Read the model definition and answer for the solid it produces. Units are mm, in the model's axes. A direction names the side the tool comes from. Coordinates: 2 decimals unless noted, no trailing zeros. Order: outer loops, then holes, each group sorted by start corner. A loop starts at its lowest first (then second) coordinate and runs counter-clockwise, first axis right, second up. Notation, with made-up numbers: (-26.75, 12) - (-7.75, 12) arc R27 cw to (-7.75, 31) - close; hole circle Ø7 at (77.25, -11). An arc over 180 degrees is marked (long way). Use one line per item in the form item = value.
```python
from build123d import *

# Parameters (mm, degrees)
BOSS_EXTRUDE1_DEPTH      = 10
SKETCH3_R                = 6.5
SKETCH3_R_2              = 4
BOSS_EXTRUDE3_DEPTH      = 7.5
SKETCH7_W                = 15
SKETCH7_H                = 12.050233058
BOSS_EXTRUDE4_DEPTH      = 10
BOSS_EXTRUDE5_DEPTH      = 10
BOSS_EXTRUDE5_DEPTH_BACK = 10
SKETCH9_R                = 6.726812024
SKETCH9_R_2              = 4.5
FILLET1_R                = 10
FILLET2_R                = 10
FILLET3_R                = 10
FILLET4_R                = 10


with BuildPart() as part:
    # Sketch1 → Boss-Extrude1 (new body)
    with BuildSketch(Plane(origin=(0, 0, 0), x_dir=(1, 0, 0), z_dir=(0, 1, 0))):
        Polygon((-11.814153955, -17.668422436), (-29.581045004, -26.851971991), (-59, -113), (-73.793817424, -113), (-41.477337097, -18.36709911), (-5.943554998, 0), (5.943554998, 0), (41.477337097, -18.36709911), (73.793817424, -113), (59, -113), (29.581045004, -26.851971991), (11.814153955, -17.668422436), align=None)
    extrude(amount=BOSS_EXTRUDE1_DEPTH)

    # Sketch3 → Boss-Extrude3 (add, symmetric)
    with BuildSketch(Plane(origin=(-66.396908712, 0, 0), x_dir=(0, 0, -1), z_dir=(1, 0, 0))):
        with Locations((-117.153311931, 5)):
            Circle(SKETCH3_R)
        with Locations((-117.153311931, 5)):
            Circle(SKETCH3_R_2, mode=Mode.SUBTRACT)
    boss_extrude3 = extrude(amount=BOSS_EXTRUDE3_DEPTH, both=True)

    # Mirror3: Boss-Extrude3 across plane
    add(boss_extrude3.mirror(Plane(origin=(0, 0, 0), x_dir=(0, 0, 1), z_dir=(1, 0, 0))))

    # Sketch7 → Boss-Extrude4 (add)
    with BuildSketch(Plane(origin=(0, 10, 0), x_dir=(1, 0, 0), z_dir=(0, 1, 0))):
        with Locations((0, 6.025116529)):
            Rectangle(SKETCH7_W, SKETCH7_H)
    extrude(amount=-BOSS_EXTRUDE4_DEPTH)

    # Sketch9 → Boss-Extrude5 (add, two sides: drawn at the far end of the back side and taken through both)
    with BuildSketch(Plane(origin=(0, 0, 0), x_dir=(0, 0, -1), z_dir=(1, 0, 0)).offset(-BOSS_EXTRUDE5_DEPTH_BACK)):
        with Locations((16.550233058, 5)):
            Circle(SKETCH9_R)
        with Locations((16.550233058, 5)):
            Circle(SKETCH9_R_2, mode=Mode.SUBTRACT)
    extrude(amount=BOSS_EXTRUDE5_DEPTH + BOSS_EXTRUDE5_DEPTH_BACK)

    # Fillet1
    # the kernel refuses this fillet: 10 mm, written as the material it adds along each edge
    with BuildSketch(Plane(origin=(-5.943554998, 0, 0), x_dir=(-0.88834455248328, 0, 0.4591774777504672), z_dir=(0, 1, 0))) as fillet1_piece_1:
        with BuildLine():
            CenterArc((5.095194407, -10), FILLET1_R, 90, 21.792944461)
            Line((1.382659439, -0.71468449), (0, 0))
            Line((0, 0), (5.095194407, 0))
        make_face()
    extrude(amount=10)

    # Fillet2
    # the kernel refuses this fillet: 10 mm, written as the material it adds along each edge
    with BuildSketch(Plane(origin=(5.943554998, 0, 0), x_dir=(0.8883445524832799, 0, 0.4591774777504676), z_dir=(0, 1, 0))) as fillet2_piece_1:
        with BuildLine():
            CenterArc((5.095194407, 10), FILLET2_R, 248.207055539, 21.792944461)
            Line((1.382659439, 0.71468449), (0, 0))
            Line((0, 0), (5.095194407, 0))
        make_face()
    extrude(amount=10)

    # Fillet3
    # the kernel refuses this fillet: 10 mm, written as the material it adds along each edge
    with BuildSketch(Plane(origin=(11.814153955, 0, 17.668422436), x_dir=(0.8883445524832799, 0, 0.4591774777504676), z_dir=(0, 1, 0)), Plane(origin=(-11.814153955, 0, 17.668422436), x_dir=(1, 0, 0), z_dir=(0, 1, 0))) as fillet3_piece_1:
        with BuildLine():
            CenterArc((FILLET3_R * 0.243164033357, -FILLET3_R), FILLET3_R, 90, 27.334044372)
            Line((-FILLET3_R * 0.216013444393, -FILLET3_R * 0.111655447517), (0, 0))
            Line((0, 0), (FILLET3_R * 0.243164033357, 0))
        make_face()
    extrude(amount=10)
    with BuildSketch(Plane(origin=(29.581045004, 0, 26.851971991), x_dir=(0.3231689910588884, 0, 0.946341272067313), z_dir=(0, 1, 0)), Plane(origin=(-29.581045004, 0, 26.851971991), x_dir=(0.8883445524832806, 0, -0.4591774777504663), z_dir=(0, 1, 0))) as fillet3_piece_2:
        with BuildLine():
            CenterArc((FILLET3_R * 0.402111719604, -FILLET3_R), FILLET3_R, 90, 43.811274916)
            Line((-FILLET3_R * 0.290173472026, -FILLET3_R * 0.278375988862), (0, 0))
            Line((0, 0), (FILLET3_R * 0.402111719604, 0))
        make_face()
    extrude(amount=10)
    with BuildSketch(Plane(origin=(-52.198620973, 10, 113), x_dir=(0, 0, -1), z_dir=(-1, 0, 0))) as fillet3_piece_3_section:
        with BuildLine():
            CenterArc((2.720551611, -10), FILLET3_R, 90, 24.619977329)
            ThreePointArc((-1.445426294, -0.909090909), (-0.692731114, -0.502215954), (0, 0))
            Line((0, 0), (2.720551611, 0))
        make_face()
    fillet3_piece_3 = extrude(amount=28.396575479, mode=Mode.PRIVATE)
    fillet3_piece_3 = split(fillet3_piece_3, bisect_by=Plane(origin=(-58.289676239, 10, 110.919946807), z_dir=(-0.9463412720673133, 0, -0.3231689910588876)), keep=Keep.TOP, mode=Mode.PRIVATE)
    fillet3_piece_3 = split(fillet3_piece_3, bisect_by=Plane(origin=(-71.538454048, 10, 106.395580932), z_dir=(0.9463412720673133, 0, 0.3231689910588875)), keep=Keep.TOP, mode=Mode.PRIVATE)
    fillet3_piece_3 = split(fillet3_piece_3, bisect_by=Plane(origin=(-73.896908712, 10, 113), z_dir=(1, 0, 0)), keep=Keep.TOP, mode=Mode.PRIVATE)
    add(fillet3_piece_3)
    with BuildSketch(Plane(origin=(80.595196452, 10, 113), x_dir=(0, 0, -1), z_dir=(-1, 0, 0))) as fillet3_piece_4_section:
        with BuildLine():
            CenterArc((2.720551611, -10), FILLET3_R, 90, 24.619977329)
            ThreePointArc((-1.445426294, -0.909090909), (-0.692731114, -0.502215954), (0, 0))
            Line((0, 0), (2.720551611, 0))
        make_face()
    fillet3_piece_4 = extrude(amount=28.396575479, mode=Mode.PRIVATE)
    fillet3_piece_4 = split(fillet3_piece_4, bisect_by=Plane(origin=(74.504141186, 10, 115.080053193), z_dir=(-0.9463412720673132, 0, 0.32316899105888797)), keep=Keep.TOP, mode=Mode.PRIVATE)
    fillet3_piece_4 = split(fillet3_piece_4, bisect_by=Plane(origin=(61.255363377, 10, 119.604419068), z_dir=(0.9463412720673132, 0, -0.32316899105888797)), keep=Keep.TOP, mode=Mode.PRIVATE)
    fillet3_piece_4 = split(fillet3_piece_4, bisect_by=Plane(origin=(73.896908712, 10, 113), z_dir=(-1, 0, 0)), keep=Keep.TOP, mode=Mode.PRIVATE)
    add(fillet3_piece_4)
    with BuildSketch(Plane(origin=(80.595196452, 0, 113), x_dir=(0, 0, -1), z_dir=(-1, 0, 0))) as fillet3_piece_5_section:
        with BuildLine():
            CenterArc((2.720551611, 10), FILLET3_R, 245.380022671, 24.619977329)
            ThreePointArc((-1.445426294, 0.909090909), (-0.692731114, 0.502215954), (0, 0))
            Line((0, 0), (2.720551611, 0))
        make_face()
    fillet3_piece_5 = extrude(amount=28.396575479, mode=Mode.PRIVATE)
    fillet3_piece_5 = split(fillet3_piece_5, bisect_by=Plane(origin=(74.504141186, 0, 115.080053193), z_dir=(-0.9463412720673132, 0, 0.32316899105888797)), keep=Keep.TOP, mode=Mode.PRIVATE)
    fillet3_piece_5 = split(fillet3_piece_5, bisect_by=Plane(origin=(61.255363377, 0, 119.604419068), z_dir=(0.9463412720673132, 0, -0.32316899105888797)), keep=Keep.TOP, mode=Mode.PRIVATE)
    fillet3_piece_5 = split(fillet3_piece_5, bisect_by=Plane(origin=(73.896908712, 0, 113), z_dir=(-1, 0, 0)), keep=Keep.TOP, mode=Mode.PRIVATE)
    add(fillet3_piece_5)
    with BuildSketch(Plane(origin=(-52.198620973, 0, 113), x_dir=(0, 0, -1), z_dir=(-1, 0, 0))) as fillet3_piece_6_section:
        with BuildLine():
            CenterArc((2.720551611, 10), FILLET3_R, 245.380022671, 24.619977329)
            ThreePointArc((-1.445426294, 0.909090909), (-0.692731114, 0.502215954), (0, 0))
            Line((0, 0), (2.720551611, 0))
        make_face()
    fillet3_piece_6 = extrude(amount=28.396575479, mode=Mode.PRIVATE)
    fillet3_piece_6 = split(fillet3_piece_6, bisect_by=Plane(origin=(-58.289676239, 0, 110.919946807), z_dir=(-0.9463412720673133, 0, -0.3231689910588876)), keep=Keep.TOP, mode=Mode.PRIVATE)
    fillet3_piece_6 = split(fillet3_piece_6, bisect_by=Plane(origin=(-71.538454048, 0, 106.395580932), z_dir=(0.9463412720673133, 0, 0.3231689910588875)), keep=Keep.TOP, mode=Mode.PRIVATE)
    fillet3_piece_6 = split(fillet3_piece_6, bisect_by=Plane(origin=(-73.896908712, 0, 113), z_dir=(1, 0, 0)), keep=Keep.TOP, mode=Mode.PRIVATE)
    add(fillet3_piece_6)
    with BuildSketch(Plane(origin=(-7.5, 10, 0), x_dir=(-0.8324412912652444, 0, 0.5541132525004725), z_dir=(0, -1, 0))) as fillet3_piece_7:
        with BuildLine():
            CenterArc((5.396772828, 9.93931012), FILLET3_R, 213.649659515, 62.665955628)
            Line((-2.927640085, 4.398177595), (-3.760081376, 3.844064343))
            Line((-3.760081376, 3.844064343), (-0.832441291, -0.554113253))
            Line((-0.832441291, -0.554113253), (-0.266857068, -0.963736118))
            ThreePointArc((-0.266857068, -0.963736118), (3.878627843, -1.295879951), (6.606829993, -0.993931012))
            Line((6.606829993, -0.993931012), (6.496824796, 0))
        make_face()
    extrude(amount=10)
    with BuildSketch(Plane(origin=(7.5, 10, 0), x_dir=(0.832441291265244, 0, 0.5541132525004732), z_dir=(0, -1, 0))) as fillet3_piece_8:
        with BuildLine():
            CenterArc((5.396772828, -9.93931012), FILLET3_R, 83.684384857, 62.665955628)
            Line((-2.927640085, -4.398177595), (-3.760081376, -3.844064343))
            Line((-3.760081376, -3.844064343), (-0.832441291, 0.554113253))
            Line((-0.832441291, 0.554113253), (-0.266857068, 0.963736118))
            ThreePointArc((-0.266857068, 0.963736118), (3.878627843, 1.295879951), (6.606829993, 0.993931012))
            Line((6.606829993, 0.993931012), (6.496824796, 0))
        make_face()
    extrude(amount=10)
    # the kernel refuses this fillet: 10 mm, written as the material it takes off along each edge
    with BuildSketch(Plane(origin=(41.477337097, -10.05279299, 18.36709911), x_dir=(0.3231689910588881, 0, 0.9463412720673132), z_dir=(0, 1, 0)), Plane(origin=(-41.477337097, -10.05279299, 18.36709911), x_dir=(0.8883445524832805, 0, -0.4591774777504667), z_dir=(0, 1, 0))) as fillet3_2_piece_1:
        with BuildLine():
            CenterArc((FILLET3_R * 0.402111719604, -FILLET3_R), FILLET3_R, 90, 43.811274916)
            Line((-FILLET3_R * 0.290173472026, -FILLET3_R * 0.278375988862), (0, 0))
            Line((0, 0), (FILLET3_R * 0.402111719604, 0))
        make_face()
    extrude(amount=30.10558598, mode=Mode.SUBTRACT)

    # Fillet4
    fillet4_edges = [part.edges().sort_by_distance(p)[0] for p in [
        (0, 10, -12.050233058),
        (0, 0, -12.050233058),
    ]]
    fillet(fillet4_edges, radius=FILLET4_R)


solid = part.part
```
(1) Section D-D, the plane x = -63 is taken. Write down the section's boundary in (y, z).
Answer list:
outline = (-0.91, 114.45) arc R10 cw to (0, 110.28) - (0, 81.39) - (10, 81.39) - (10, 110.28) arc R10 cw to (10.91, 114.45) arc R6.5 ccw (long way) to start; hole circle Ø8 at (5, 117.15)
(2) Straight lines are drawn through the part: L1, parallel to Y at x = 44, z = 59; L2, parallel to Z at x = -3.75, y = 5; L3, parallel to X at y = 9, z = 86.5. For each, find the intervals that lie inside material, in ascending order.
Answer list:
L1 = 0 to 10
L2 = -23.28 to -21.05, -12.05 to 17.67
L3 = -64.74 to -49.95, 49.95 to 64.74
(3) Section B-B, the plane z = 50 is taken. Write down the section's boundary in (x, y), then the cut area to 3 significant figures.
Answer list:
outline = (-52.28, 0) - (-37.49, 0) - (-37.49, 10) - (-52.28, 10) - close; (37.49, 0) - (52.28, 0) - (52.28, 10) - (37.49, 10) - close
area = 296 mm2
(4) Given pin 1 Ø5 at (y, z) = (5, 117.15) entering from +X; pin 2 Ø2.5 at (y, z) = (4.5, -10) entering from -X; pin 3 Ø3.5 at (y, z) = (6.5, 120) entering from -X; pin 4 Ø3 at (y, z) = (5.5, 91.5) entering from +X, each flat-ended and moving along its own axis, determine where each tip first touches the part or whether it passes through.
Answer list:
pin_1 = through
pin_2 = -10
pin_3 = -73.9
pin_4 = 66.96
(5) The mould has two halves that part along X. Classify faces 4 (the flat face through (58.897, 5, 122)), 5 (the flat face through (3, 10, 17)), 6 (the flat face through (-10, 7, -21)): +X half, -X half, draft (parallel to the pull), parting line (faces both ways), or undercut.
Answer list:
face_4 = undercut
face_5 = draft
face_6 = -X half
(6) Section A-A, the plane x = 3.5 is taken. Write down the section's boundary in (y, z), then the cut area to 3 significant figures.
Answer list:
outline = (-1.03, -13.57) arc R6.73 ccw (long way) to (11.03, -13.57) arc R10 cw to (10, -9.15) - (10, 17.67) - (0, 17.67) - (0, -9.15) arc R10 cw to start; hole circle Ø9 at (5, -16.55)
area = 362 mm2
(7) Section C-C, the plane y = 5 is taken. State how many separate pieces and enclosed holes the cut face has, then the cut area to 3 significant figures.
Answer list:
separate_pieces = 4
enclosed_holes = 0
area = 4,100 mm2
(8) Which of the six approach directions +Z, -Z, +X, -X, +Y, -Y give full straight-line access (tool end or side, diameter ignored) to faces 1 (the cylindrical face through (-28.957, 4.93, 27.32)), 2 (the cylindrical face through (66.095, -0.236, 112.441)), 3 (the flat face through (3, 0, 17))?
Answer list:
face_1 = +Z, +Y, -Y
face_2 = -Z, +X, -X, -Y
face_3 = +X, -X, -Y
